Check sheet for the modelled part. Datum: model origin and axes. Units: mm. A direction names the side the tool comes from. Round coordinates to 2 decimals unless told otherwise and drop trailing zeros. Loops run counter-clockwise (first coordinate to the right, second up) from the corner with the lowest first, then second, coordinate; pieces in that order, holes last. Notation, with made-up numbers: (19, 3.25) - (70, 3.25) arc R31 cw to (70, 42.25) - close; hole circle Ø8 at (-38, -28.5). An arc over 180 degrees is marked (long way). Answer in a Markdown table with one row per item. Add a question column.
(1) Thickness scan on line 1 along X through (y, z) = (2.4, 1); line 2 along Y through (x, z) = (11.25, -1); line 3 along Z through (x, y) = (4.25, 3.6). Record the ranges inside material, lowest first.
(2) Cross-section at A-A on x = -9. Enter the section's corners in (y, z), then the cut area to 3 significant figures.
(3) Access from +Z, -Z, +X, -X, +Y, -Y to the whole of each face (thin tool, end or side, straight path). Record for faces 1 (the flat face through (-7.7, 3.05, 8.5)), 2 (the flat face through (-7.8, 2.5, 8.5)), 3 (the flat face through (-5.5, 3, 7)), 4 (the flat face through (-10, 3, 7)), 5 (the flat face through (-8, 3, 5.5)).
(4) Cross-section at D-D on x = 2.75. Enter the section's corners in (y, z), then the cut area to 3 significant figures.
(5) Cross-section at B-B on z = 0.25. Enter the section's corners in (x, y), then the cut area to 3 significant figures.
(6) Gauge pin test, flat ends, axial feed: pin 1 (5 mm diameter, centred on x = -0.5, z = -4, fed in from +Y); pin 2 (1.4 mm diameter, centred on x = 6.5, y = 3.5, fed in from -Z); pin 3 (1.4 mm diameter, centred on x = 4.5, y = 3.5, fed in from +Z). Record the tip position at first contact, or that the pin passes through.
(7) Cross-section at C-C on y = 1.4. Enter the section's corners in (x, z).
Autodesk Inventor part; units mm, degrees
ref_plane "YZ Plane" through (0, 0, 0) normal (1, 0, 0) x (0, 1, 0)
ref_plane "XZ Plane" through (0, 0, 0) normal (0, 1, 0) x (-1, 0, 0)
ref_plane "XY Plane" through (0, 0, 0) normal (0, 0, 1) x (1, 0, 0)
sketch "Sketch1" plane through (0, 0, 0) normal (0, 1, 0) x (-1, 0, 0)
  line L0 (-13, 8) -> (13, 8)
  line L1 (13, 8) -> (13, -8)
  line L2 (13, -8) -> (-13, -8)
  line L3 (-13, -8) -> (-13, 8)
  line L4 (-13, 8) -> (13, -8) construction
  line L5 (13, 8) -> (-13, -8) construction
  point P0 (0, 0)
  dimension "d0" = 26
  dimension "d1" = 16
extrude "Extrusion1" add sketch "Sketch1" along normal blind 2
sketch "Sketch2" plane through (0, 2, 0) normal (0, 1, 0) x (1, 0, 0)
  line L0 (13, -8) -> (13, 8) construction
  line L1 (13, 8) -> (-13, 8) construction
  line L2 (-13, 8) -> (-13, -8) construction
  line L3 (-13, -8) -> (13, -8) construction
  line L4 (-13, 8) -> (-13, -8) construction
  line L5 (-13, -8) -> (-10, -8) construction
  line L6 (-13, -8) -> (13, -8) construction
  line L7 (-10, -8) -> (-10, -5.5)
  line L8 (-10, -5.5) -> (-5.5, -5.5)
  line L9 (-5.5, -5.5) -> (-5.5, -8)
  line L10 (-5.5, -8) -> (-10, -8)
  point P0 (0, 0)
  dimension "d4" = 3
  dimension "d5" = 2.5
  dimension "d6" = 4.5
extrude "Extrusion2" add sketch "Sketch2" along normal blind 1.55
sketch "Sketch3" plane through (-13, 0, 8) normal (0, 0, 1) x (1, 0, 0)
  line L0 (0, 0) -> (26, 0) construction
  line L1 (26, 0) -> (26, 2) construction
  line L2 (7.5, 2) -> (26, 2) construction
  line L3 (7.5, 2) -> (7.5, 3.55) construction
  line L4 (3, 3.55) -> (7.5, 3.55) construction
  line L5 (3, 2) -> (3, 3.55) construction
  line L6 (0, 2) -> (3, 2) construction
  line L7 (0, 0) -> (0, 2) construction
  line L8 (3, 3.55) -> (7.5, 3.55) construction
  line L9 (7.5, 3.55) -> (7.5, 2) construction
  line L10 (7.5, 2) -> (3, 2) construction
  line L11 (3, 2) -> (3, 3.55) construction
  line L12 (3.5, 2.5) -> (7, 2.5)
  line L13 (7, 2.5) -> (7, 3.05)
  line L14 (7, 3.05) -> (3.5, 3.05)
  line L15 (3.5, 3.05) -> (3.5, 2.5)
  point P0 (13, 0)
  dimension "d9" = 0.5
extrude "Extrusion3" add sketch "Sketch3" along normal blind 1
sketch "Sketch4" plane through (0, 2, 0) normal (0, 1, 0) x (1, 0, 0)
  line L0 (13, -8) -> (13, 8) construction
  line L1 (13, -8) -> (8.428, -8) construction
  line L2 (-13, -8) -> (13, -8) construction
  line L3 (8.428, -8) -> (8.428, -4.952) construction
  line L4 (8.428, -4.952) -> (2.0526, -4.952)
  line L5 (2.0526, -4.952) -> (2.0526, 1.652)
  line L6 (2.0526, 1.652) -> (8.428, 1.652)
  line L7 (8.428, 1.652) -> (8.428, -4.952)
  point P0 (0, 0)
  dimension "d12" = 4.572
  dimension "d13" = 3.048
  dimension "d14" = 6.3754
  dimension "d15" = 6.604
extrude "Extrusion4" add sketch "Sketch4" along normal blind 2.794
properties part number "BMS"
Answers:
| question | item | result |
|---|---|---|
| 1 | line 1 | x = 2.05 to 8.43 |
| 1 | line 2 | y = 0 to 2 |
| 1 | line 3 | z = -1.65 to 4.95 |
| 2 | outline | (0, -8) - (2, -8) - (2, 5.5) - (3.55, 5.5) - (3.55, 8) - (3.05, 8) - (3.05, 9) - (2.5, 9) - (2.5, 8) - (0, 8) - close |
| 2 | area | 36.4 mm^2 |
| 3 | face 1 | +Z, +X, -X, +Y |
| 3 | face 2 | +Z, +X, -X, -Y |
| 3 | face 3 | +Z, -Z, +X, +Y |
| 3 | face 4 | +Z, -Z, -X, +Y |
| 3 | face 5 | -Z, +X, -X, +Y |
| 4 | outline | (0, -8) - (2, -8) - (2, -1.65) - (4.79, -1.65) - (4.79, 4.95) - (2, 4.95) - (2, 8) - (0, 8) - close |
| 4 | area | 50.5 mm^2 |
| 5 | outline | (-13, 0) - (13, 0) - (13, 2) - (8.43, 2) - (8.43, 4.79) - (2.05, 4.79) - (2.05, 2) - (-13, 2) - close |
| 5 | area | 69.8 mm^2 |
| 6 | pin 1 | stops at y = 2 |
| 6 | pin 2 | stops at z = -1.65 |
| 6 | pin 3 | stops at z = 4.95 |
| 7 | outline | (-13, -8) - (13, -8) - (13, 8) - (-13, 8) - close |
